Design review of the part shown in the three views and the two pictorial views. Dimensions are in mm from the part's minimum x, y and z. A direction names the side the tool comes from. Give positions to 0.01 mm unless a question says otherwise; leave off trailing zeros. Write each loop counter-clockwise with the first axis right and the second up, starting at its lowest first coordinate (ties: lowest second). Pieces come first, ordered by that corner, then holes. Notation, with made-up numbers: M 69,2.25 L 75,2.25 A12 cw 75,22.25 Z; hole C 83.5,7 d9. An arc over 180 degrees is marked long. Use one line per item in the form item = value. Start each with the question number.
Q1. For probe 1 along X at (y, z) = (73.4, 8); probe 2 along Z at (x, y) = (1, 25); probe 3 along X at (y, z) = (48, 10.5), list the stretches that pass through material, from the lowest coordinate up. Write a range as [from, to].
Q2. Clearance check with a flat-ended pin moving along its axis: pin 1 Ø4 at (x, y) = (28, 44) entering from +Z. State where the tip first meets the part, or that it passes through.
Q3. Tool access review of the marked faces 4 and 5: name each direction out of +Z, -Z, +X, -X, +Y, -Y from which nothing blocks a thin tool from reaching the whole face with its end or side.
Q4. Consider section D-D on y = 10.5. Write out the cut boundary in (x, z), and give its area (3 significant figures).
Q5. Mouldability with a two-part tool opening along Y and no side actions: class the marked faces 1, 2 and 3 as released by +Y, released by -Y, zero draft, split by the parting line, or undercut.
Q6. Consider section A-A on y = 25. Write out the cut boundary in (x, z), and give its area (3 significant figures).
Q7. Consider section B-B on z = 4. Write out the cut boundary in (x, y), and give its area (3 significant figures).
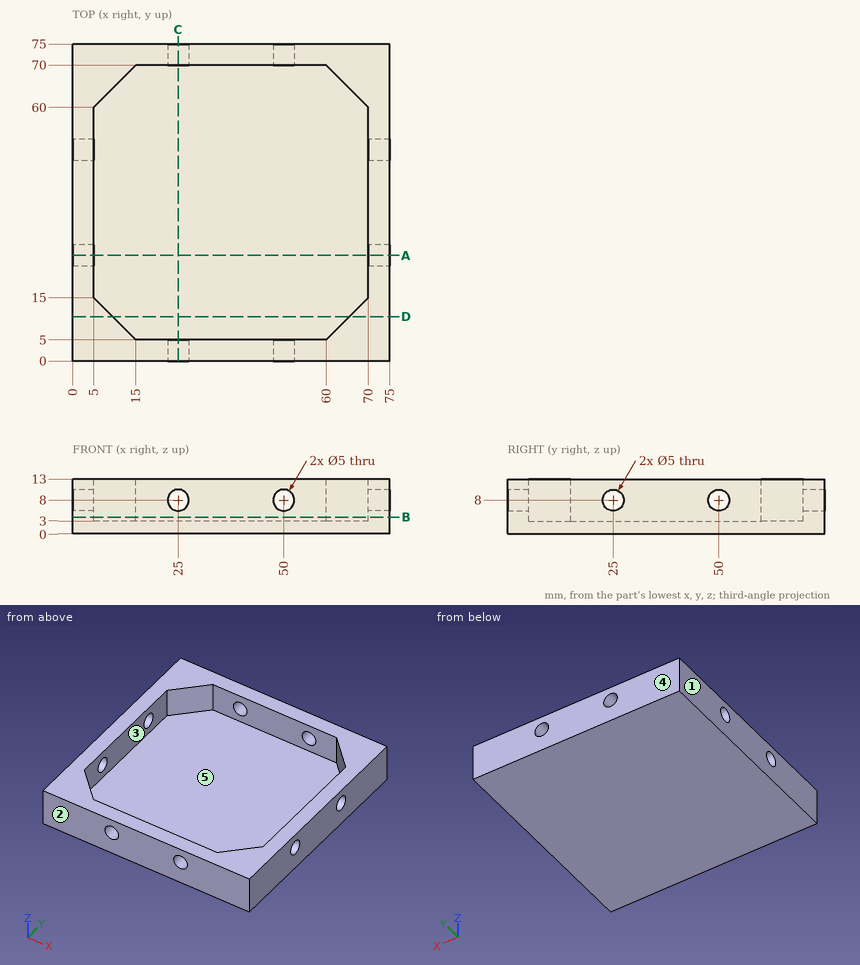
Working result:
q1.probe_1 = [0, 22.5], [27.5, 47.5], [52.5, 75]
q1.probe_2 = [0, 5.5], [10.5, 13]
q1.probe_3 = [0, 5], [70, 75]
q2.pin_1 = 3
q3.face_4 = +Z, -Z, +X, -X, +Y
q3.face_5 = +Z
q4.outline = M 0,0 L 75,0 L 75,13 L 65.5,13 L 65.5,3 L 9.5,3 L 9.5,13 L 0,13 Z
q4.area = 415 mm²
q5.face_1 = zero draft
q5.face_2 = released by -Y
q5.face_3 = undercut
q6.outline = M 0,0 L 75,0 L 75,5.5 L 70,5.5 L 70,3 L 5,3 L 5,5.5 L 0,5.5 Z; M 0,10.5 L 5,10.5 L 5,13 L 0,13 Z; M 70,10.5 L 75,10.5 L 75,13 L 70,13 Z
q6.area = 275 mm²
q7.outline = M 0,0 L 75,0 L 75,75 L 0,75 Z; hole M 5,15 L 15,5 L 60,5 L 70,15 L 70,60 L 60,70 L 15,70 L 5,60 Z
q7.area = 1,600 mm²
